For this review, take the finished solid that the model builds, in its own axes (mm). A direction names the side the tool comes from. Round coordinates to 2 decimals unless told otherwise and drop trailing zeros. Write each loop counter-clockwise with the first axis right and the second up, starting at its lowest first coordinate (ties: lowest second). Pieces come first, ordered by that corner, then holes. Notation, with made-up numbers: M -25,-30.75 L 24,-30.75 A28 ccw 24,0.25 Z; hole C 69,45 d10. An arc over 180 degrees is marked long. Use one line per item in the form item = value. Start each with the question number.
Item 1: Add section B-B (x = 4). State the section outline as (y, z) points.
Item 2: Add section A-A (z = -4). State the section outline as (x, y) points, and give its area (3 significant figures).
Item 3: Add section D-D (z = -1.25). State the section outline as (x, y) points, and give its area (3 significant figures).
Item 4: For line 1 (X direction, y = 3.8, z = -4); line 2 (Z direction, x = -4, y = 2.3); line 3 (X direction, y = 1.05, z = -16), list the stretches that pass through material, from the lowest coordinate up. Write a range as [from, to].
Item 5: For faces 1 (the cylindrical face through (-2.614, 1.479, -15.425)), 2 (the flat face through (8, 4.5, -9.9)), list the 3-axis set-ups (+Z, -Z, +X, -X, +Y, -Y) from which the entire face can be reached by the end or side of a thin tool; tool diameter is ignored.
Item 6: For P1, Ø9, axis at x = -3.5, z = -5.5, coming from the +Y side; P2, Ø0.8, axis at y = 4.5, z = -13.5, coming from the -X side; P3, Ø0.5, axis at y = 3.5, z = -11.5, coming from the -X side, all flat-tipped, find the tip position at first contact; note any pin that passes through.
Item 7: Add section C-C (y = 2). Count the separate pieces of the cut face and the enclosed holes in it, and give its area (3 significant figures).
Item 8: Draft analysis for pull direction Z (two halves, no side actions). For faces 3 (the flat face through (10, 5, -10)), 4 (the flat face through (6, 2, -20)), 5 (the cylindrical face through (5.48, 1.97, -3.39)), 6 (the cylindrical face through (10.4, 2.46, -4.07)), state which applies: released by +Z, released by -Z, zero draft, split by the parting line, or undercut.
from build123d import *

# Parameters (mm, degrees)
SKETCH1_W           = 8
SKETCH1_H           = 20
SKETCH1_R           = 1.55
SKETCH1_R_2         = 1.5
SKETCH1_R_3         = 1.6
BOSS_EXTRUDE7_DEPTH = 5
SKETCH1_8_W         = 8
SKETCH1_8_H         = 20
SKETCH1_8_R         = 1.6
SKETCH1_8_R_2       = 1.55
SKETCH1_8_R_3       = 1.5
BOSS_EXTRUDE8_DEPTH = 4
SKETCH1_9_W         = 8
SKETCH1_9_H         = 20
SKETCH1_9_R         = 1.6
SKETCH1_9_R_2       = 1.55
SKETCH1_9_R_3       = 1.5
BOSS_EXTRUDE9_DEPTH = 3


with BuildPart() as part:
    # Sketch1 → Boss-Extrude7 (new body)
    with BuildSketch(Plane(origin=(0, 0, 0), x_dir=(1, 0, 0), z_dir=(0, 1, 0))):
        with Locations((12, 10)):
            Rectangle(SKETCH1_W, SKETCH1_H)
        with Locations((12, 10)):
            Circle(SKETCH1_R, mode=Mode.SUBTRACT)
        with Locations((12, 16)):
            Circle(SKETCH1_R_2, mode=Mode.SUBTRACT)
        with Locations((12, 4)):
            Circle(SKETCH1_R_3, mode=Mode.SUBTRACT)
    extrude(amount=BOSS_EXTRUDE7_DEPTH)

    # Sketch1_8 → Boss-Extrude8 (add)
    with BuildSketch(Plane(origin=(0, 0, 0), x_dir=(1, 0, 0), z_dir=(0, 1, 0))):
        with Locations((4, 10)):
            Rectangle(SKETCH1_8_W, SKETCH1_8_H)
        with Locations((4, 4)):
            Circle(SKETCH1_8_R, mode=Mode.SUBTRACT)
        with Locations((4, 10)):
            Circle(SKETCH1_8_R_2, mode=Mode.SUBTRACT)
        with Locations((4, 16)):
            Circle(SKETCH1_8_R_3, mode=Mode.SUBTRACT)
    extrude(amount=BOSS_EXTRUDE8_DEPTH)

    # Sketch1_9 → Boss-Extrude9 (add)
    with BuildSketch(Plane(origin=(0, 0, 0), x_dir=(1, 0, 0), z_dir=(0, 1, 0))):
        with Locations((-4, 10)):
            Rectangle(SKETCH1_9_W, SKETCH1_9_H)
        with Locations((-4, 4)):
            Circle(SKETCH1_9_R, mode=Mode.SUBTRACT)
        with Locations((-4, 10)):
            Circle(SKETCH1_9_R_2, mode=Mode.SUBTRACT)
        with Locations((-4, 16)):
            Circle(SKETCH1_9_R_3, mode=Mode.SUBTRACT)
    extrude(amount=BOSS_EXTRUDE9_DEPTH)


solid = part.part
Calculated:
q1.outline = M 0,-20 L 4,-20 L 4,-17.5 L 0,-17.5 Z; M 0,-14.5 L 4,-14.5 L 4,-11.55 L 0,-11.55 Z; M 0,-8.45 L 4,-8.45 L 4,-5.6 L 0,-5.6 Z; M 0,-2.4 L 4,-2.4 L 4,0 L 0,0 Z
q2.outline = M -8,0 L -5.6,0 L -5.6,3 L -8,3 Z; M -2.4,0 L 2.4,0 L 2.4,4 L 0,4 L 0,3 L -2.4,3 Z; M 5.6,0 L 10.4,0 L 10.4,5 L 8,5 L 8,4 L 5.6,4 Z; M 13.6,0 L 16,0 L 16,5 L 13.6,5 Z
q2.area = 57.6 mm^2
q3.outline = M -8,0 L 16,0 L 16,5 L 8,5 L 8,4 L 0,4 L 0,3 L -8,3 Z
q3.area = 96.0 mm^2
q4.line_1 = [0, 2.4], [5.6, 10.4], [13.6, 16]
q4.line_2 = [-20, -17.5], [-14.5, -11.55], [-8.45, -5.6], [-2.4, 0]
q4.line_3 = [-8, -5.5], [-2.5, 2.5], [5.5, 10.5], [13.5, 16]
q5.face_1 = +Y, -Y
q5.face_2 = +Z, -Z, -X, +Y
q6.P1 = 4
q6.P2 = 8
q6.P3 = 0
q7.separate_pieces = 1
q7.enclosed_holes = 9
q7.area = 412 mm^2
q8.face_3 = zero draft
q8.face_4 = released by -Z
q8.face_5 = undercut
q8.face_6 = undercut
